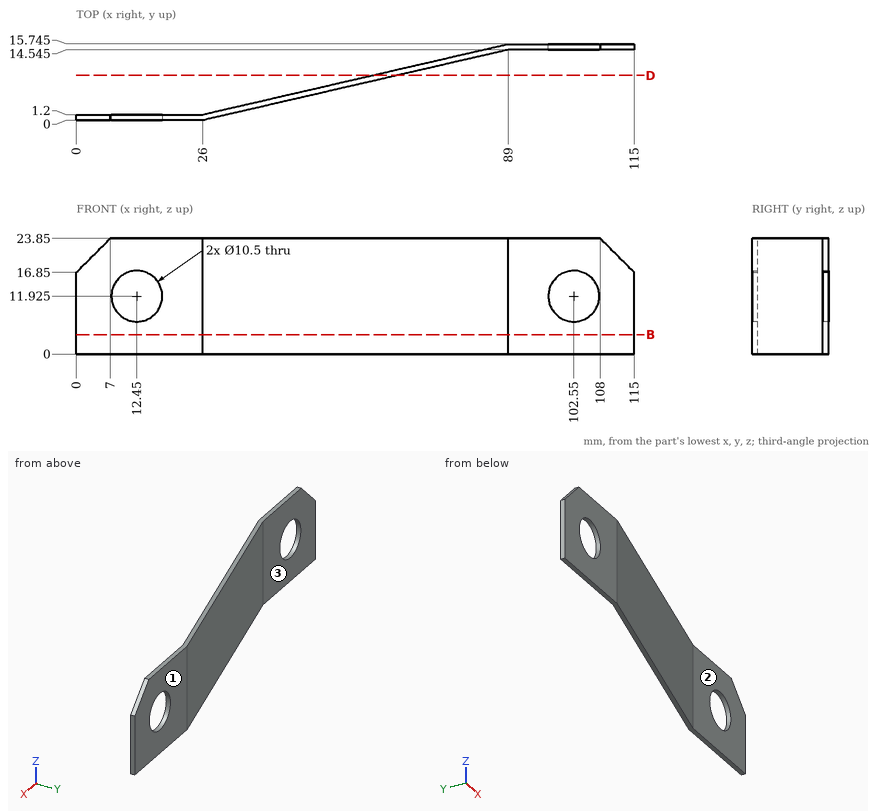
Can you work these out from the drawing? Everything is in mm from the part's minimum corner. A direction names the side the tool comes from. Give positions to 0.01 mm unless a question says otherwise; leave off trailing zeros. Write each loop counter-clockwise with the first axis right and the second up, starting at its lowest first coordinate (ties: lowest second). Pieces come first, ordered by that corner, then holes. Notation, with made-up numbers: (-27, 5) -> (28, 5) arc R20 ccw to (28, 25) -> close; hole circle Ø5 at (25, 21.25). An arc over 180 degrees is marked (long way). Write each question's results on one line, items separated by ' | '. Start each with the question number.
Q1. Which directions (+Z, -Z, +X, -X, +Y, -Y) give clear straight access to the entire face, cutting with the end or side of a thin tool? Please do the marked faces 1, 2 and 3.
Q2. I'm going to push flat-ended pins straight in: pin 1 Ø5 at (x, z) = (47, 14.5) entering from +Y (1 decimal); pin 2 Ø4 at (x, z) = (28.5, 13.5) entering from -Y (1 decimal); pin 3 Ø12 at (x, z) = (9.5, 12) entering from +Y; pin 4 Ø3 at (x, y) = (29, 4.5) entering from -Z. Where does each tip first touch, or does it pass through?
Q3. I need wall thicknesses on probe 1 along Y at (x, z) = (98.5, 21.5) (1 decimal); probe 2 along Y at (x, z) = (6, 20.25). Which ranges of each line are inside material? Lowest first, please.
Q4. Suppose I cut it at D-D, the plane y = 9.25. List the corners of the cut face in (x, z) for me, and give its area (3 significant figures).
Q5. Suppose I cut it at B-B, the plane z = 4. List the corners of the cut face in (x, y) for me (1 decimal).
Outcome:
1) face 1: +Z, -Z, +X, -X, +Y | face 2: +Z, -Z, +X, -Y | face 3: +Z, -Z, -X, +Y
2) pin 1: y = 6.6 | pin 2: y = 0.1 | pin 3: y = 1.2 | pin 4: through
3) probe 1: 14.5 to 15.7 | probe 2: 0 to 1.2
4) outline: (60.87, 0) -> (66.07, 0) -> (66.07, 23.85) -> (60.87, 23.85) -> close | area: 124 mm2
5) outline: (0, 0) -> (26, 0) -> (89, 14.5) -> (115, 14.5) -> (115, 15.7) -> (89, 15.7) -> (26, 1.2) -> (0, 1.2) -> close
